```python
from build123d import *

# Parameters (mm, degrees)
F0_R     = 12.7
F1_DEPTH = 6.35
F3_D     = 6.35
F4_SIZE  = 3.175


with BuildPart() as f1:
    # F0 (on Right) → F1 (new body)
    with BuildSketch(Plane.YZ):
        Circle(F0_R)
    extrude(amount=-F1_DEPTH)

    # F3 (through all)
    with Locations(Plane.YZ):
        with Locations((0, 0)):
            Hole(F3_D / 2)

    # F4
    f4_edges = [f1.edges().sort_by_distance(p)[0] for p in [
        (-6.35, -12.7, 0),
    ]]
    chamfer(f4_edges, length=F4_SIZE)


solid = f1.part
```
Here's how the part is built. I have some questions about the finished solid (model axes, mm). Give positions to 0.01 mm unless a question says otherwise; leave off trailing zeros. Order: outer loops, then holes, each group sorted by start corner. A loop starts at its lowest first (then second) coordinate and runs counter-clockwise, first axis right, second up. Notation, with made-up numbers: M -31,61.25 L 1,61.25 A24 ccw 1,72.25 Z; hole C 35,-37.75 d8. An arc over 180 degrees is marked long. Use a Markdown table: item, result. Add a question column.
1. If we mould it in two halves opening along Z, with no side actions, what happens to faces 1 (the cylindrical face through (-1.57, -2.75, -12.4)), 2 (the cylindrical face through (-3.22, 0.69, -3.1)), 3 (the flat face through (-6.35, 4, 0))? For each: +Z half, -Z half, draft (parallel to the pull), parting line (faces both ways), or undercut.
2. I need wall thicknesses on probe 1 along Z at (x, y) = (-2.5, 0) (3 decimals); probe 2 along X at (y, z) = (1.25, 11.5); probe 3 along Z at (x, y) = (-4.75, -3.75). Which ranges of each line are inside material? Lowest first, please. Write a range as from..to.
3. Suppose I cut it at A-A (z = 0). List the corners of the cut face in (x, y) for me (3 decimals).
4. Suppose I cut it at D-D (x = -3.5). List the corners of the cut face in (y, z) for me (3 decimals), and give its area (3 significant figures).
5. Suppose I cut it at C-C (x = -0.5). List the corners of the cut face in (y, z) for me (3 decimals).
6. For pin 1 Ø2 at (x, y) = (-5.5, -5) entering from +Z, with a flat end and sliding along its axis, tell me the tip position at first contact or that it passes through.
Results list:
| question | item | result |
|---|---|---|
| 1 | face 1 | parting line |
| 1 | face 2 | undercut |
| 1 | face 3 | draft |
| 2 | probe 1 | z = -12.7..-3.175, 3.175..12.7 |
| 2 | probe 2 | x = -4.31..0 |
| 2 | probe 3 | z = -10.47..10.47 |
| 3 | outline | M -6.35,-9.525 L -3.175,-12.7 L 0,-12.7 L 0,-3.175 L -6.35,-3.175 Z; M -6.35,3.175 L 0,3.175 L 0,12.7 L -3.175,12.7 L -6.35,9.525 Z |
| 4 | outline | C 0,0 d24.75; hole C 0,0 d6.35 |
| 4 | area | 449 mm² |
| 5 | outline | C 0,0 d25.4; hole C 0,0 d6.35 |
| 6 | pin 1 | stops at z = 10.31 |
